Read the model definition and answer for the solid it produces. Units are mm, in the model's axes. Round coordinates to 2 decimals unless told otherwise and drop trailing zeros. Order: outer loops, then holes, each group sorted by start corner. A loop starts at its lowest first (then second) coordinate and runs counter-clockwise, first axis right, second up. Notation, with made-up numbers: (81.25, 43) - (127.25, 43) arc R19 cw to (127.25, 68) - close; hole circle Ø10 at (74, -38.75). An arc over 180 degrees is marked (long way). Put each result on its own line as item: value. Start each with the question number.
Q1. Section A-A on z = 1.25 is taken. State how many separate pieces and enclosed holes the cut face has, then the cut area to 3 significant figures.
Q2. Find the intervals of material crossed by line 1 along X through (y, z) = (18, 4.75); line 2 along Y through (x, z) = (29, 7.75); line 3 along X through (y, z) = (-1.5, 0.75), in increasing order. Write a range as from..to.
Q3. Section B-B on y = 79 is taken. Give the vertices of the cut face in (x, z).
Q4. Section D-D on y = 49.5 is taken. Give the vertices of the cut face in (x, z).
Q5. Each of these flat-tipped pins is pushed along its axis until it touches: pin 1 Ø4 at (x, z) = (36.5, 5) entering from +Y; pin 2 Ø4 at (y, z) = (90.5, 3.5) entering from -X; pin 3 Ø2.5 at (x, z) = (-53.5, 5) entering from -Y; pin 4 Ø1 at (x, y) = (-13.5, 29) entering from -Z. Where does it stop, or does it pass through?
Q6. Section C-C on x = 6.5 is taken. Give the vertices of the cut face in (y, z), then the cut area to 3 significant figures.
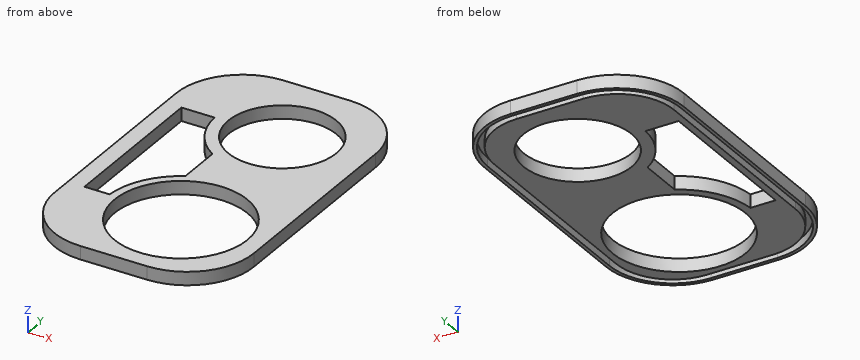
from build123d import *

# Parameters (mm, degrees)
F0_R     = 40
F0_R_2   = 32.5
F1_DEPTH = 8
F2_DEPTH = 5


with BuildPart() as f1:
    # F0 (on Top) → F1 (new body)
    with BuildSketch(Plane.XY):
        with BuildLine():
            Line((9.88816, 113.519735), (-30.11184, 113.519735))
            ThreePointArc((-30.11184, 113.519735), (-58.396111, 101.804006), (-70.11184, 73.519735))
            Line((-70.11184, 73.519735), (-70.11184, -46.480265))
            ThreePointArc((-70.11184, -46.480265), (-58.396111, -74.764536), (-30.11184, -86.480265))
            Line((-30.11184, -86.480265), (9.88816, -86.480265))
            ThreePointArc((9.88816, -86.480265), (38.172431, -74.764536), (49.88816, -46.480265))
            Line((49.88816, -46.480265), (49.88816, 73.519735))
            ThreePointArc((49.88816, 73.519735), (38.172431, 101.804006), (9.88816, 113.519735))
        make_face()
        with BuildLine():
            ThreePointArc((-68.11184, 73.519735), (-56.981898, 100.389793), (-30.11184, 111.519735))
            Line((-30.11184, 111.519735), (9.88816, 111.519735))
            ThreePointArc((9.88816, 111.519735), (36.758217, 100.389793), (47.88816, 73.519735))
            Line((47.88816, 73.519735), (47.88816, -46.480265))
            ThreePointArc((47.88816, -46.480265), (36.758217, -73.350323), (9.88816, -84.480265))
            Line((9.88816, -84.480265), (-30.11184, -84.480265))
            ThreePointArc((-30.11184, -84.480265), (-56.981898, -73.350323), (-68.11184, -46.480265))
            Line((-68.11184, -46.480265), (-68.11184, 73.519735))
        make_face(mode=Mode.SUBTRACT)
        with BuildLine():
            Line((9.88816, 111.519735), (-30.11184, 111.519735))
            ThreePointArc((-30.11184, 111.519735), (-56.981898, 100.389793), (-68.11184, 73.519735))
            Line((-68.11184, 73.519735), (-68.11184, -46.480265))
            ThreePointArc((-68.11184, -46.480265), (-56.981898, -73.350323), (-30.11184, -84.480265))
            Line((-30.11184, -84.480265), (9.88816, -84.480265))
            ThreePointArc((9.88816, -84.480265), (36.758217, -73.350323), (47.88816, -46.480265))
            Line((47.88816, -46.480265), (47.88816, 73.519735))
            ThreePointArc((47.88816, 73.519735), (36.758217, 100.389793), (9.88816, 111.519735))
        make_face()
        with BuildLine():
            Line((-64.11184, -46.480265), (-64.11184, 73.519735))
            ThreePointArc((-64.11184, 73.519735), (-54.153471, 97.561365), (-30.11184, 107.519735))
            Line((-30.11184, 107.519735), (9.88816, 107.519735))
            ThreePointArc((9.88816, 107.519735), (33.92979, 97.561365), (43.88816, 73.519735))
            Line((43.88816, 73.519735), (43.88816, -46.480265))
            ThreePointArc((43.88816, -46.480265), (33.92979, -70.521896), (9.88816, -80.480265))
            Line((9.88816, -80.480265), (-30.11184, -80.480265))
            ThreePointArc((-30.11184, -80.480265), (-54.153471, -70.521896), (-64.11184, -46.480265))
        make_face(mode=Mode.SUBTRACT)
        with BuildLine():
            ThreePointArc((-30.11184, 107.519735), (-54.153471, 97.561365), (-64.11184, 73.519735))
            Line((-64.11184, 73.519735), (-64.11184, -46.480265))
            ThreePointArc((-64.11184, -46.480265), (-54.153471, -70.521896), (-30.11184, -80.480265))
            Line((-30.11184, -80.480265), (9.88816, -80.480265))
            ThreePointArc((9.88816, -80.480265), (33.92979, -70.521896), (43.88816, -46.480265))
            Line((43.88816, -46.480265), (43.88816, 73.519735))
            ThreePointArc((43.88816, 73.519735), (33.92979, 97.561365), (9.88816, 107.519735))
            Line((9.88816, 107.519735), (-30.11184, 107.519735))
        make_face()
        with Locations((-0.11184, -36.480265)):
            Circle(F0_R, mode=Mode.SUBTRACT)
        with BuildLine():
            Line((-60.095887, 62.39015), (-40.095887, 62.39015))
            ThreePointArc((-40.095887, 62.39015), (-34.900309, 43.777332), (-21.585297, 29.772281))
            Line((-21.585297, 29.772281), (-21.585297, 3.065792))
            ThreePointArc((-21.585297, 3.065792), (-37.93282, -12.096388), (-44.995373, -33.24476))
            Line((-44.995373, -33.24476), (-60.095887, -33.24476))
            Line((-60.095887, -33.24476), (-60.095887, 62.39015))
        make_face(mode=Mode.SUBTRACT)
        with Locations((-0.11184, 63.519735)):
            Circle(F0_R_2, mode=Mode.SUBTRACT)
    extrude(amount=F1_DEPTH)

    # F0 (on Top) → F2 (cut)
    with BuildSketch(Plane.XY):
        with BuildLine():
            Line((9.88816, 111.519735), (-30.11184, 111.519735))
            ThreePointArc((-30.11184, 111.519735), (-56.981898, 100.389793), (-68.11184, 73.519735))
            Line((-68.11184, 73.519735), (-68.11184, -46.480265))
            ThreePointArc((-68.11184, -46.480265), (-56.981898, -73.350323), (-30.11184, -84.480265))
            Line((-30.11184, -84.480265), (9.88816, -84.480265))
            ThreePointArc((9.88816, -84.480265), (36.758217, -73.350323), (47.88816, -46.480265))
            Line((47.88816, -46.480265), (47.88816, 73.519735))
            ThreePointArc((47.88816, 73.519735), (36.758217, 100.389793), (9.88816, 111.519735))
        make_face()
        with BuildLine():
            Line((-64.11184, -46.480265), (-64.11184, 73.519735))
            ThreePointArc((-64.11184, 73.519735), (-54.153471, 97.561365), (-30.11184, 107.519735))
            Line((-30.11184, 107.519735), (9.88816, 107.519735))
            ThreePointArc((9.88816, 107.519735), (33.92979, 97.561365), (43.88816, 73.519735))
            Line((43.88816, 73.519735), (43.88816, -46.480265))
            ThreePointArc((43.88816, -46.480265), (33.92979, -70.521896), (9.88816, -80.480265))
            Line((9.88816, -80.480265), (-30.11184, -80.480265))
            ThreePointArc((-30.11184, -80.480265), (-54.153471, -70.521896), (-64.11184, -46.480265))
        make_face(mode=Mode.SUBTRACT)
    extrude(amount=F2_DEPTH, mode=Mode.SUBTRACT)


solid = f1.part
Findings:
1. separate pieces: 2
1. enclosed holes: 4
1. area: 9,420 mm2
2. line 1: -70.11..-68.11, -64.11..-60.1, -21.59..43.89, 47.89..49.89
2. line 2: -81.62..-63.91, -9.05..49.07, 77.97..108.66
2. line 3: -70.11..-68.11, -64.11..-60.1, -28.42..-19.51, 19.29..43.89, 47.89..49.89
3. outline: (-69.73, 0) - (-67.71, 0) - (-67.71, 5) - (-63.67, 5) - (-63.67, 0) - (-28.69, 0) - (-28.69, 8) - (-69.73, 8) - close; (28.46, 0) - (43.44, 0) - (43.44, 5) - (47.49, 5) - (47.49, 0) - (49.51, 0) - (49.51, 8) - (28.46, 8) - close
4. outline: (-70.11, 0) - (-68.11, 0) - (-68.11, 5) - (-64.11, 5) - (-64.11, 0) - (-60.1, 0) - (-60.1, 8) - (-70.11, 8) - close; (-37.57, 0) - (-29.43, 0) - (-29.43, 8) - (-37.57, 8) - close; (29.21, 0) - (43.89, 0) - (43.89, 5) - (47.89, 5) - (47.89, 0) - (49.89, 0) - (49.89, 8) - (29.21, 8) - close
5. pin 1: y = 105.05
5. pin 2: x = -67.2
5. pin 3: y = -79.8
5. pin 4: z = 0
6. outline: (-86.48, 0) - (-84.48, 0) - (-84.48, 5) - (-80.48, 5) - (-80.48, 0) - (-75.93, 0) - (-75.93, 8) - (-86.48, 8) - close; (2.97, 0) - (31.7, 0) - (31.7, 8) - (2.97, 8) - close; (95.34, 0) - (107.52, 0) - (107.52, 5) - (111.52, 5) - (111.52, 0) - (113.52, 0) - (113.52, 8) - (95.34, 8) - close
6. area: 420 mm2
